Input: part model. Units: mm. Frame: model coordinates. A direction names the side the tool comes from. Round coordinates to 2 decimals unless told otherwise and drop trailing zeros. Order: outer loops, then holes, each group sorted by start corner. A loop starts at its lowest first (then second) coordinate and runs counter-clockwise, first axis right, second up.
Item 1: Cut plane D-D on x = 6. Output: boundary loops of the cut face in (y, z), then the cut area to 3 significant figures.
Item 2: Reachability of faces 4 (the flat face through (13, 0, 49.8)), 5 (the flat face through (0, 3, 51.8)), 6 (the cylindrical face through (-0.571, 2.226, 44.812)) from +Z, -Z, +X, -X, +Y, -Y: full face, straight path, thin tool, end or side. Return the list, or none.
Item 3: Line query: L1, parallel to Z at x = 0, y = 1.25; L2, parallel to X at y = 1, z = 55; L3, parallel to Z at x = 0, y = 2.25. Output: solid intervals per line, ascending.
Item 4: First-contact query: pin 1 (4.5 mm diameter, centred on x = -12.5, z = 55, fed in from +Y); pin 2 (6 mm diameter, centred on x = -2.5, z = 16, fed in from -Y); pin 3 (1.1 mm diameter, centred on x = -0.5, z = 43, fed in from +Y); pin 4 (3 mm diameter, centred on x = -7, y = 2.5, fed in from +Z). Flat tips, straight axial feed; report the tip coordinate or a pass-through.
Item 5: Cut plane C-C on y = 3.25. Output: boundary loops of the cut face in (x, z), then the cut area to 3 significant figures.
Item 6: Cut plane A-A on z = 43. Output: boundary loops of the cut face in (x, y).
Item 7: Cut plane B-B on x = 12.5. Output: boundary loops of the cut face in (y, z), then the cut area to 3 significant figures.
Item 8: Mould query, pull axis X, two halves, no side actions, for faces 1 (the flat face through (0.2, 0.5, -2)), 2 (the cylindrical face through (-12.57, 0.42, 56.7)), 3 (the cylindrical face through (-16.68, -0.03, 50.4)). Classes: released by +X, released by -X, zero draft, split by the parting line, or undercut.
Autodesk Inventor part; units mm, degrees
ref_plane "YZ Plane" through (0, 0, 0) normal (1, 0, 0) x (0, 1, 0)
ref_plane "XZ Plane" through (0, 0, 0) normal (0, 1, 0) x (-1, 0, 0)
ref_plane "XY Plane" through (0, 0, 0) normal (0, 0, 1) x (1, 0, 0)
sketch "Skizze1" plane through (0, 0, 0) normal (0, 1, 0) x (-1, 0, 0)
  line L0 (17.75, 60) -> (-17.75, 60)
  line L1 (-17.75, 60) -> (-17.75, 0)
  line L2 (-17.75, 0) -> (17.75, 0)
  line L3 (17.75, 0) -> (17.75, 60)
  point P0 (0, 0)
  point P1 (0, 0)
  dimension "d0" = 60
  dimension "d1" = 35.5
extrude "Extrusion1" add sketch "Skizze1" along normal blind 2
sketch "Skizze3" plane through (0, 2, 0) normal (0, 1, 0) x (1, 0, 0)
  line L0 (-17.75, 0) -> (-17.75, -60)
  line L1 (17.75, -60) -> (17.75, 0)
  line L2 (-17.75, -51.8) -> (17.75, -51.8)
  line L3 (17.75, -51.8) -> (17.75, -6.2)
  line L4 (-17.75, -6.2) -> (-17.75, -51.8)
  line L5 (17.75, 0) -> (-17.75, 0)
  line L6 (-17.75, -6.2) -> (17.75, -6.2)
  point P0 (0, 0)
  point P1 (17.75, -51.8)
  point P2 (0, 0)
  dimension "d71" = 51.8
  dimension "d75" = 6.2
extrude "Extrusion3" add sketch "Skizze3" along normal blind 2 contours L6 L1 L2 L0
sketch "Skizze6" plane through (0, 0, 0) normal (0, -1, 0) x (1, 0, 0)
  line L0 (-17.75, 60) -> (17.75, 60)
  line L1 (11.25, 60) -> (-11.25, 60)
  line L2 (-11.25, 60) -> (-11.25, 0)
  line L3 (-11.25, 0) -> (11.25, 0)
  line L4 (11.25, 0) -> (11.25, 60)
  line L5 (8.65, 60) -> (-8.65, 60)
  line L6 (-8.65, 60) -> (-8.65, 0)
  line L7 (-8.65, 0) -> (8.65, 0)
  line L8 (8.65, 0) -> (8.65, 60)
  line L9 (0, -15.6) -> (0, 72.6)
  line L10 (17.75, 0) -> (-17.75, 0)
  point P0 (0, 0)
  point P1 (0, 60)
  point P2 (0, -1)
  point P3 (0, 60)
  point P4 (0, 0)
  point P5 (8.65, 0)
  point P6 (-8.65, 0)
  dimension "d24" = 17.3
  dimension "d25" = 22.5
extrude "Extrusion6" add sketch "Skizze6" along normal blind 2 contours L0 L6 L3 L2 | L0 L4 L3 L8
sketch "Skizze7" plane through (0, -2, 0) normal (0, -1, 0) x (1, 0, 0)
  line L0 (17.75, 0) -> (11.25, 0)
  line L1 (11.25, 0) -> (11.25, 60)
  line L2 (11.25, 60) -> (17.75, 60)
  line L3 (17.75, 60) -> (17.75, 0)
  point P0 (0, 0)
  dimension "d31" = 6.5
extrude "Extrusion7" cut sketch "Skizze7" against normal through all
mirror "Spiegeln2" about plane through (0, 0, 0) normal (1, 0, 0) of "Extrusion7"
sketch "Skizze9" plane through (0, 0, 0) normal (0, -1, 0) x (1, 0, 0)
  line L0 (0, -12) -> (0, 72)
  line L1 (-11.25, 51.8) -> (-11.25, 60)
  line L2 (11.25, 6.2) -> (11.25, 0)
  line L3 (-11.25, 60) -> (11.25, 60)
  line L4 (11.25, 51.8) -> (-11.25, 51.8)
  line L5 (11.25, 60) -> (11.25, 51.8)
  line L6 (-11.25, 0) -> (-11.25, 6.2)
  line L7 (-11.25, 6.2) -> (11.25, 6.2)
  line L8 (11.25, 0) -> (-11.25, 0)
  point P0 (0, 0)
  point P1 (0, 3)
  point P2 (0, 0)
  dimension "d79" = 3
hole "Bohrung1" at (0, 0, 3) direction (0, 1, 0) diameter 3.4 depth 4
sketch "Skizze10" plane through (0, 4, 0) normal (0, 1, 0) x (1, 0, 0)
  line L0 (0, 12) -> (0, -72)
  circle A0 centre (0, -3) radius 1.7
  point P0 (0, 0)
  point P1 (0, -43)
  dimension "d46" = 40
hole "Bohrung2" at (0, 4, 43) direction (0, -1, 0) diameter 3.4 depth 4 counterbore diameter 3.8 counterbore depth 3.5
sketch "Skizze11" plane through (-11.25, 4, 9.2) normal (-1, 0, 0) x (0, 0, 1)
  line L0 (50.8, -6) -> (42.6, -6)
  line L1 (42.6, -6) -> (42.6, -2)
  line L2 (42.6, -2) -> (50.8, -2)
  line L3 (50.8, -2) -> (50.8, -6)
  point P0 (-9.2, -4)
  point P1 (42.6, -2)
extrude "Extrusion9" add sketch "Skizze11" along normal blind 6
sketch "Skizze12" plane through (0, -2, 0) normal (0, -1, 0) x (1, 0, 0)
  line L0 (-8.65, 60) -> (-17.25, 60)
  line L1 (-11.25, 51.8) -> (-11.25, 0)
  line L2 (-11.25, 51.8) -> (-17.25, 51.8)
  point P0 (0, 0)
  point P1 (-12.5, 55)
  point P2 (-11.25, 9.2)
  dimension "d80" = 1.25
  dimension "d81" = 3.2
hole "Bohrung3" at (-12.5, -2, 55) direction (0, 1, 0) diameter 3.4 depth 4 countersink diameter 5 countersink angle 90
sketch "Skizze13" plane through (-11.25, -2, 51.8) normal (0, 0, -1) x (-1, 0, 0)
  line L0 (0, 0) -> (0, 4)
  line L1 (0, 0) -> (6, 0)
  line L2 (6, 4) -> (6, 0)
  line L3 (0, 4) -> (6, 4)
  point P0 (-11.25, 2)
extrude "Extrusion10" add sketch "Skizze13" along normal blind 2
fillet "Rundung1" radius 2 2 edges at (-17.25, 0, 60) (-17.25, 0, 49.8)
mirror "Spiegeln6" about plane through (0, 0, 0) normal (1, 0, 0) of "Extrusion9", "Bohrung3", "Extrusion10", "Rundung1"
chamfer "Fasen3" distance 1 angle 45 2 edges at (-8.65, -2, 30) (8.65, -2, 30)
sketch "Skizze14" plane through (8.65, 0, 0) normal (0, 0, -1) x (-1, 0, 0)
  line L0 (0, -1) -> (-1, -2)
  line L1 (0, 0) -> (0, -1)
  line L2 (0, 0) -> (17.3, 0)
  line L3 (17.3, 0) -> (17.3, -1)
  line L4 (18.3, -2) -> (17.3, -1)
  line L5 (19.9, -2) -> (18.3, -2)
  line L6 (19.9, -2) -> (19.9, 2)
  line L7 (-2.6, 2) -> (19.9, 2)
  line L8 (-2.6, 2) -> (-2.6, -2)
  line L9 (-1, -2) -> (-2.6, -2)
  point P0 (8.65, 0)
extrude "Extrusion11" add sketch "Skizze14" along normal blind 2
properties part number "Zwischenplatte"
From the geometry:
1. outline: (0, -2) - (2, -2) - (2, 6.2) - (4, 6.2) - (4, 51.8) - (2, 51.8) - (2, 60) - (0, 60) - close
1. area: 215 mm2
2. face 4: -Z, +X, +Y, -Y
2. face 5: +Z, +X, -X, +Y
2. face 6: +Y
3. L1: z = -2 to 1.3, 4.7 to 41.1, 44.9 to 60
3. L2: x = -17.25 to -14.2, -10.8 to 10.8, 14.2 to 17.25
3. L3: z = 6.2 to 41.1, 44.9 to 51.8
4. pin 1: stops at y = 2
4. pin 2: stops at y = 0
4. pin 3: passes through
4. pin 4: stops at z = 60
5. outline: (-11.25, 6.2) - (11.25, 6.2) - (11.25, 51.8) - (-11.25, 51.8) - close; hole circle Ø3.8 at (0, 43)
5. area: 1,010 mm2
6. outline: (-11.25, -2) - (-9.65, -2) - (-8.65, -1) - (-8.65, 0) - (-1.7, 0) - (-1.7, 0.5) - (-1.9, 0.5) - (-1.9, 4) - (-11.25, 4) - close; (1.7, 0) - (8.65, 0) - (8.65, -1) - (9.65, -2) - (11.25, -2) - (11.25, 4) - (1.9, 4) - (1.9, 0.5) - (1.7, 0.5) - close
7. outline: (-2, 49.8) - (2, 49.8) - (2, 53.3) - (-1.2, 53.3) - (-2, 52.5) - close; (-2, 57.5) - (-1.2, 56.7) - (2, 56.7) - (2, 60) - (-2, 60) - close
7. area: 26.6 mm2
8. face 1: zero draft
8. face 2: undercut
8. face 3: released by -X
